from build123d import *

# Parameters (mm, degrees)
F0_R     = 12.7
F1_DEPTH = 6.35
F2_R     = 1.524
F3_W     = 6.35
F3_H     = 69.85
F5_R     = 12.7
F5_R_2   = 4.7625
F6_DEPTH = 6.35


with BuildPart() as f1:
    # F0 (on Top) → F1 (new body)
    with BuildSketch(Plane.XY):
        with BuildLine():
            Line((-50.8, -19.05), (50.8, -19.05))
            Line((50.8, -19.05), (50.8, -9.652))
            Line((50.8, -9.652), (35.052, -9.652))
            ThreePointArc((35.052, -9.652), (25.4, 0), (35.052, 9.652))
            Line((35.052, 9.652), (50.8, 9.652))
            Line((50.8, 9.652), (50.8, 19.05))
            Line((50.8, 19.05), (-50.8, 19.05))
            Line((-50.8, 19.05), (-50.8, 9.652))
            Line((-50.8, 9.652), (-35.052, 9.652))
            ThreePointArc((-35.052, 9.652), (-25.4, 0), (-35.052, -9.652))
            Line((-35.052, -9.652), (-50.8, -9.652))
            Line((-50.8, -9.652), (-50.8, -19.05))
        make_face()
        Circle(F0_R, mode=Mode.SUBTRACT)
    extrude(amount=F1_DEPTH)

    # F2
    f2_edges = [f1.edges().sort_by_distance(p)[0] for p in [
        (-50.8, 19.05, 3.175),
        (50.8, 19.05, 3.175),
        (50.8, -19.05, 3.175),
        (-50.8, -19.05, 3.175),
    ]]
    fillet(f2_edges, radius=F2_R)

    # F3 (on Right) → F4 (revolve)
    with BuildSketch(Plane.YZ):
        with Locations((-15.875, -34.925)):
            Rectangle(F3_W, F3_H)
    revolve(axis=Axis((0, 0, -16.966719), (0, 0, -1)))

    # F5 (on face) → F6 (join)
    with BuildSketch(Plane(origin=(0, 0, -69.85), x_dir=(1, 0, 0), z_dir=(0, 0, -1))):
        Circle(F5_R)
        Circle(F5_R_2, mode=Mode.SUBTRACT)
    extrude(amount=-F6_DEPTH)


solid = f1.part
Design review of the part built by this model. Coordinates are the model's own, in mm. A direction names the side the tool comes from. Give positions to 0.01 mm unless a question says otherwise; leave off trailing zeros. Order: outer loops, then holes, each group sorted by start corner. A loop starts at its lowest first (then second) coordinate and runs counter-clockwise, first axis right, second up. Notation, with made-up numbers: (20, -32.75) - (55, -32.75) arc R20 ccw to (55, -16.75) - close; hole circle Ø1 at (88.5, 45.25). An arc over 180 degrees is marked (long way). Use CSV: the item, a comma, the result in double quotes. Start each with the question number.
Q1. Take a section at B-B (x = 37.5). State the section outline as (y, z) points, and give its area (3 significant figures).
Q2. Draft analysis for pull direction Y (two halves, no side actions). For faces 5 (the face through (-25.402, 0.212, 3.131)), 6 (the face through (-50.8, 14, 3)), 7 (the face through (-1, -19.05, 3)), state which applies: pulls with the +Y half, pulls with the -Y half, needs draft (parallel to the pull), parting line crosses it, or undercut.
Q3. Take a section at A-A (y = 0). State the section outline as (x, z) points.
Q4. For line 1 (Y direction, x = 0, z = -67.5); line 2 (X direction, y = 0, z = 3.5); line 3 (Y direction, x = 0, z = -22), list the stretches that pass through material, from the lowest coordinate up.
Q5. For P1, Ø20.5, axis at x = 0, y = 0, coming from the +Z side; P2, Ø3, axis at y = -11, z = -53, coming from the +X side; P3, Ø5, axis at x = 9, z = -13.5, coming from the -Y side; P4, Ø7.5, axis at x = 0, y = 0, coming from the +Z side, all flat-tipped, find the tip position at first contact; note any pin that passes through.
Q6. Machinability: for faces 1 (the face through (5, 0, -63.5)), 2 (the face through (-43, 9.652, 3)), 3 (the face through (43, 9.652, 3)), 4 (the face through (11.59, 15.12, -34.44)), which of the approach directions +Z, -Z, +X, -X, +Y, -Y give a long, thin tool a straight path to every point of the face, cutting with its end or side? Answer none if there is none.
Q7. Take a section at C-C (z = -35). State the section outline as (x, y) points, and give its area (3 significant figures).
Q8. Take a section at D-D (y = -15.5). State the section outline as (x, z) points.
Calculated:
1,outline,"(-19.05, 0) - (-9.65, 0) - (-9.65, 6.35) - (-19.05, 6.35) - close; (9.65, 0) - (19.05, 0) - (19.05, 6.35) - (9.65, 6.35) - close"
1,area,"119 mm²"
2,face 5,"undercut"
2,face 6,"needs draft"
2,face 7,"pulls with the -Y half"
3,outline,"(-25.4, 0) - (-19.05, 0) - (-19.05, -69.85) - (-4.76, -69.85) - (-4.76, -63.5) - (-12.7, -63.5) - (-12.7, 6.35) - (-25.4, 6.35) - close; (4.76, -69.85) - (19.05, -69.85) - (19.05, 0) - (25.4, 0) - (25.4, 6.35) - (12.7, 6.35) - (12.7, -63.5) - (4.76, -63.5) - close"
4,line 1,"y = -19.05 to -4.76, 4.76 to 19.05"
4,line 2,"x = -25.4 to -12.7, 12.7 to 25.4"
4,line 3,"y = -19.05 to -12.7, 12.7 to 19.05"
5,P1,"stops at z = -63.5"
5,P2,"stops at x = 16.51"
5,P3,"stops at y = -17.91"
5,P4,"passes through"
6,face 1,"+Z"
6,face 2,"+Z, -Z, -X"
6,face 3,"+Z, -Z, +X"
6,face 4,"-Z"
7,outline,"circle Ø38.1 at (0, 0); hole circle Ø25.4 at (0, 0)"
7,area,"633 mm²"
8,outline,"(-50.8, 0) - (-11.07, 0) - (-11.07, -69.85) - (11.07, -69.85) - (11.07, 0) - (50.8, 0) - (50.8, 6.35) - (-50.8, 6.35) - close"
